Design review of the part built by this model. Coordinates are the model's own, in mm. A direction names the side the tool comes from. Round coordinates to 2 decimals unless told otherwise and drop trailing zeros. Order: outer loops, then holes, each group sorted by start corner. A loop starts at its lowest first (then second) coordinate and runs counter-clockwise, first axis right, second up. Notation, with made-up numbers: (65, 59.5) - (100, 59.5) arc R18 cw to (100, 68.5) - close; hole circle Ø11 at (-23, -16.5). An arc over 180 degrees is marked (long way). Use CSV: the item, a comma, the result in double quotes.
Autodesk Inventor part; units mm, degrees
ref_plane "YZ Plane" through (0, 0, 0) normal (1, 0, 0) x (0, 1, 0)
ref_plane "XZ Plane" through (0, 0, 0) normal (0, 1, 0) x (-1, 0, 0)
ref_plane "XY Plane" through (0, 0, 0) normal (0, 0, 1) x (1, 0, 0)
sketch "Sketch1" plane through (0, 0, 0) normal (0, 1, 0) x (-1, 0, 0)
  line L0 (0, 0) -> (-79.375, 0)
  line L1 (-79.375, 0) -> (-79.375, 38.1)
  line L2 (-79.375, 38.1) -> (0, 38.1)
  line L3 (0, 38.1) -> (0, 0)
  dimension "d0" = 79.375
  dimension "d1" = 38.1
extrude "Extrusion1" add sketch "Sketch1" along normal blind 3.175
sketch "Sketch2" plane through (0, 3.175, 0) normal (0, 1, 0) x (1, 0, 0)
  line L0 (0, 0) -> (0, -38.1)
  line L1 (79.375, -38.1) -> (79.375, 0)
  line L2 (0, -33.3121) -> (79.375, -33.3121)
  line L3 (79.375, -33.3121) -> (79.375, -36.5125)
  line L4 (79.375, -36.5125) -> (0, -36.5125)
  line L5 (0, -36.5125) -> (0, -33.3121)
  line L6 (0, -38.1) -> (79.375, -38.1)
  line L7 (79.375, 0) -> (0, 0)
  line L8 (79.375, -3.175) -> (0, -3.175)
  line L9 (0, -3.175) -> (0, -6.604)
  line L10 (0, -6.604) -> (79.375, -6.604)
  line L11 (79.375, -6.604) -> (79.375, -3.175)
  dimension "d4" = 3.2004
  dimension "d8" = 1.5875
  dimension "d13" = 3.175
  dimension "d14" = 3.429
extrude "Extrusion2" cut sketch "Sketch2" against normal blind 1.5875 contours L8 L1 L10 L0 | L2 L1 L4 L0
sketch "Sketch4" plane through (0, 3.175, 0) normal (0, 1, 0) x (1, 0, 0)
  line L0 (0, -33.3121) -> (79.375, -33.3121)
  line L1 (79.375, -33.3121) -> (79.375, -6.604)
  line L2 (25.781, -21.0566) -> (34.925, -21.0566)
  line L3 (34.925, -21.0566) -> (34.925, -24.6126)
  line L4 (34.925, -24.6126) -> (25.781, -24.6126)
  line L5 (25.781, -24.6126) -> (25.781, -21.0566)
  line L6 (46.99, -14.7701) -> (73.025, -14.7701)
  line L7 (73.025, -14.7701) -> (73.025, -26.2001)
  line L8 (73.025, -26.2001) -> (46.99, -26.2001)
  line L9 (46.99, -26.2001) -> (46.99, -14.7701)
  point P0 (0, 0)
  dimension "d15" = 3.556
  dimension "d16" = 9.144
  dimension "d17" = 8.6995
  dimension "d18" = 44.45
  dimension "d19" = 26.035
  dimension "d20" = 11.43
  dimension "d21" = 7.112
  dimension "d22" = 6.35
extrude "Extrusion4" cut sketch "Sketch4" against normal blind 25.4
fillet "Fillet1" radius 1.5875 4 edges at (25.781, 1.5875, 21.0566) (25.781, 1.5875, 24.6126) (34.925, 1.5875, 24.6126) (34.925, 1.5875, 21.0566)
fillet "Fillet2" radius 1.5875 4 edges at (73.025, 1.5875, 14.7701) (73.025, 1.5875, 26.2001) (46.99, 1.5875, 26.2001) (46.99, 1.5875, 14.7701)
properties part number "Electronics Container Part 2"
1) Insertion check: pin 1 Ø1.6 at (x, z) = (50, 34.5) entering from +Y. The pin has a flat end and moves straight along its axis. Give the tip position at first contact, or say it passes through.
Data:
pin 1,"stops at y = 1.59"
2) We need section C-C (x = 13). Give the boundary of the cut face in (y, z) (1 decimal), then the cut area to 3 significant figures.
Data:
outline,"(0, 0) - (3.2, 0) - (3.2, 3.2) - (1.6, 3.2) - (1.6, 6.6) - (3.2, 6.6) - (3.2, 33.3) - (1.6, 33.3) - (1.6, 36.5) - (3.2, 36.5) - (3.2, 38.1) - (0, 38.1) - close"
area,"110 mm2"
3) We need section A-A (y = 2.45). Give the number of separate pieces and of enclosed holes in the cut face, then the cut area to 3 significant figures.
Data:
separate pieces,"3"
enclosed holes,"2"
area,"2,170 mm2"
4) We need section B-B (x = 68.5). Give the boundary of the cut face in (y, z) (1 decimal).
Data:
outline,"(0, 0) - (3.2, 0) - (3.2, 3.2) - (1.6, 3.2) - (1.6, 6.6) - (3.2, 6.6) - (3.2, 14.8) - (0, 14.8) - close; (0, 26.2) - (3.2, 26.2) - (3.2, 33.3) - (1.6, 33.3) - (1.6, 36.5) - (3.2, 36.5) - (3.2, 38.1) - (0, 38.1) - close"
5) To check wall thickness, follow L1, parallel to Z at x = 24, y = 1.95 (1 decimal); L2, parallel to X at y = 2.8, z = 23 (3 decimals); L3, parallel to Z at x = 65, y = 0.35. State the ranges of each line that lie inside material, in increasing order. Write a range as from..to.
Data:
L1,"z = 0..3.2, 6.6..33.3, 36.5..38.1"
L2,"x = 0..25.781, 34.925..46.99, 73.025..79.375"
L3,"z = 0..14.77, 26.2..38.1"
6) For faces 5 (the face through (34.45, 1.57, 21.51)), 6 (the face through (39, 2, 0)), 7 (the face through (39, 2, 6.604)), list the 3-axis set-ups (+Z, -Z, +X, -X, +Y, -Y) from which the entire face can be reached by the end or side of a thin tool; tool diameter is ignored.
Data:
face 5,"+Y, -Y"
face 6,"-Z, +X, -X, +Y, -Y"
face 7,"+X, -X, +Y"
7) We need section D-D (z = 35). Give the boundary of the cut face in (x, y) (1 decimal).
Data:
outline,"(0, 0) - (79.4, 0) - (79.4, 1.6) - (0, 1.6) - close"
8) The part is to be moulded in two halves that separate along Z. For faces 1 (the face through (39, 1.588, 35)), 2 (the face through (40, 2, 38.1)), 3 (the face through (40, 3.175, 2)), 4 (the face through (47.47, 1.57, 25.75)), say which applies: +Z half, -Z half, draft (parallel to the pull), parting line (faces both ways), or undercut.
Data:
face 1,"undercut"
face 2,"+Z half"
face 3,"draft"
face 4,"undercut"
